Part model, mm, in its own coordinate system. Face numbers are marked on the shaded views. A direction names the side the tool comes from. Coordinates: 2 decimals unless noted, no trailing zeros. Loops run counter-clockwise (first coordinate to the right, second up) from the corner with the lowest first, then second, coordinate; pieces in that order, holes last. Notation, with made-up numbers: (76.25, 82.5) -> (81.25, 82.5) arc R16 ccw to (81.25, 87.5) -> close; hole circle Ø7 at (-13, 48.5). An arc over 180 degrees is marked (long way). One line per item, written item: value. Start each with the question number.
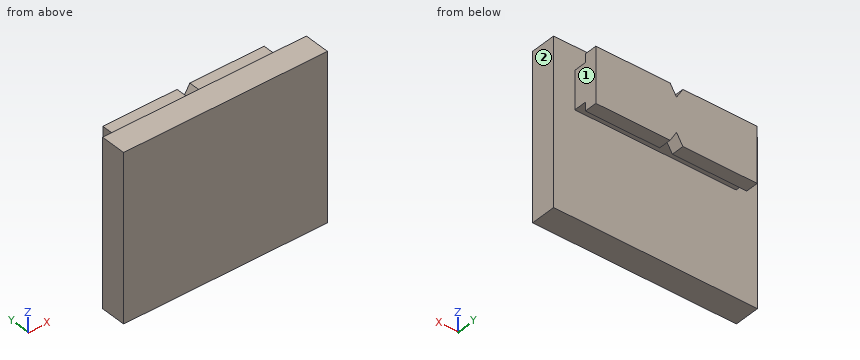
from build123d import *

# Parameters (mm, degrees)
SKETCH1_W           = 24
SKETCH1_H           = 19.5
BOSS_EXTRUDE1_DEPTH = 3
SKETCH3_W           = 19
SKETCH3_H           = 4.5
BOSS_EXTRUDE2_DEPTH = 1.5
SKETCH4_W           = 19
SKETCH4_H           = 6.5
BOSS_EXTRUDE3_DEPTH = 1.5
CUT_EXTRUDE1_DEPTH  = 1.5


with BuildPart() as part:
    # Sketch1 → Boss-Extrude1 (new body)
    with BuildSketch(Plane(origin=(0, 0, 0), x_dir=(1, 0, 0), z_dir=(0, 1, 0))):
        Rectangle(SKETCH1_W, SKETCH1_H)
    extrude(amount=BOSS_EXTRUDE1_DEPTH)

    # Sketch3 → Boss-Extrude2 (add)
    with BuildSketch(Plane(origin=(0, 3, 0), x_dir=(1, 0, 0), z_dir=(0, 1, 0))):
        with Locations((0, -4.8)):
            Rectangle(SKETCH3_W, SKETCH3_H)
    extrude(amount=BOSS_EXTRUDE2_DEPTH)

    # Sketch4 → Boss-Extrude3 (add)
    with BuildSketch(Plane(origin=(0, 4.5, 0), x_dir=(1, 0, 0), z_dir=(0, 1, 0))):
        with Locations((0, -4.8)):
            Rectangle(SKETCH4_W, SKETCH4_H)
    extrude(amount=BOSS_EXTRUDE3_DEPTH)

    # Sketch5 → Cut-Extrude1 (cut)
    with BuildSketch(Plane(origin=(0, 6, 0), x_dir=(1, 0, 0), z_dir=(0, 1, 0))):
        Polygon((0, -2.8), (0.75, -1.55), (-0.75, -1.55), align=None)
        Polygon((0, -6.8), (0.75, -8.05), (-0.75, -8.05), align=None)
    extrude(amount=-CUT_EXTRUDE1_DEPTH, mode=Mode.SUBTRACT)


solid = part.part
1) Slice it at B-B (y = 5.05). Give the cut face in (x, z), then the cut area to 3 significant figures.
2) Slice it at D-D (x = 8). Give the cut face in (y, z).
3) Pin check, flat tips, straight feed: pin 1 Ø1.5 at (x, z) = (6, 0) entering from +Y; pin 2 Ø0.8 at (x, y) = (7, 5.5) entering from -Z; pin 3 Ø1.2 at (x, y) = (7, 5.5) entering from +Z. Stop position of each tip, or through.
4) Slice it at A-A (z = 2.25). Give the cut face in (x, y).
5) Probe line 1 (Y direction, x = 9.5, z = -1); line 2 (Z direction, x = -1, y = 4.25); line 3 (Z direction, x = 5, y = 5.5). List the from-to ranges inside material, lowest first. Write a range as from..to.
6) Tool access for the marked faces 1 and 2: list every direction of +Z, -Z, +X, -X, +Y, -Y with a clear straight run to the whole face (end or side of a thin tool).
7) Slice it at C-C (z = 5). Give the cut face in (x, y).
Check sheet entries:
1. outline: (-9.5, 1.55) -> (-0.75, 1.55) -> (0, 2.8) -> (0.75, 1.55) -> (9.5, 1.55) -> (9.5, 8.05) -> (0.75, 8.05) -> (0, 6.8) -> (-0.75, 8.05) -> (-9.5, 8.05) -> close
1. area: 122 mm^2
2. outline: (0, -9.75) -> (3, -9.75) -> (3, 2.55) -> (4.5, 2.55) -> (4.5, 1.55) -> (6, 1.55) -> (6, 8.05) -> (4.5, 8.05) -> (4.5, 7.05) -> (3, 7.05) -> (3, 9.75) -> (0, 9.75) -> close
3. pin 1: stops at y = 3
3. pin 2: stops at z = 1.55
3. pin 3: stops at z = 8.05
4. outline: (-12, 0) -> (12, 0) -> (12, 3) -> (-12, 3) -> close; (-9.5, 4.5) -> (-0.33, 4.5) -> (-0.33, 6) -> (-9.5, 6) -> close; (0.33, 4.5) -> (9.5, 4.5) -> (9.5, 6) -> (0.33, 6) -> close
5. line 1: y = 0..3
5. line 2: z = 2.55..7.05
5. line 3: z = 1.55..8.05
6. face 1: +Z, -Z, +X, +Y
6. face 2: +Z, -Z, +X, +Y, -Y
7. outline: (-12, 0) -> (12, 0) -> (12, 3) -> (9.5, 3) -> (9.5, 6) -> (-9.5, 6) -> (-9.5, 3) -> (-12, 3) -> close
